```python
from build123d import *

# Parameters (mm, degrees)
SKETCH_R           = 1
SKETCH_W           = 78.96
SKETCH_H           = 50.34
PAD_DEPTH          = 5
SKETCH001_W        = 74.96
SKETCH001_H        = 46.34
PAD001_DEPTH       = 2
SKETCH002_R        = 3
SKETCH002_R_2      = 1
PAD002_DEPTH       = 10
PAD003_DEPTH       = 50
SKETCH004_W        = 40
SKETCH004_H        = 4
POCKET_DEPTH       = 57.001
POCKET_DEPTH_BACK  = -57.001
SKETCH005_R        = 1.5
POCKET001_DEPTH    = 322.817597
POLARPATTERN_COUNT = 4


with BuildPart() as part:
    # Sketch → Pad (new body)
    with BuildSketch(Plane.XY):
        with BuildLine():
            Line((-42.48, 28.17), (-3, 28.17))
            ThreePointArc((3, 28.17), (0, 31.17), (-3, 28.17))
            Line((3, 28.17), (42.48, 28.17))
            Line((42.48, 28.17), (42.48, 3))
            ThreePointArc((42.48, -3), (45.48, 0), (42.48, 3))
            Line((42.48, -3), (42.48, -28.17))
            Line((3, -28.17), (42.48, -28.17))
            ThreePointArc((-3, -28.17), (0, -31.17), (3, -28.17))
            Line((-42.48, -28.17), (-3, -28.17))
            Line((-42.48, -3), (-42.48, -28.17))
            ThreePointArc((-42.48, 3), (-45.48, 0), (-42.48, -3))
            Line((-42.48, 28.17), (-42.48, 3))
        make_face()
        with Locations((42.48, 0)):
            Circle(SKETCH_R, mode=Mode.SUBTRACT)
        with Locations((0, -28.17)):
            Circle(SKETCH_R, mode=Mode.SUBTRACT)
        with Locations((-42.48, 0)):
            Circle(SKETCH_R, mode=Mode.SUBTRACT)
        with Locations((0, 28.17)):
            Circle(SKETCH_R, mode=Mode.SUBTRACT)
        Rectangle(SKETCH_W, SKETCH_H, mode=Mode.SUBTRACT)
    extrude(amount=PAD_DEPTH)

    # Sketch001 → Pad001 (join)
    with BuildSketch(Plane.XY):
        with BuildLine():
            Line((-57, 23.235), (-57, -23.235))
            ThreePointArc((-57, -23.235), (-53.338835, -32.073835), (-44.5, -35.735))
            Line((-44.5, -35.735), (44.5, -35.735))
            ThreePointArc((44.5, -35.735), (53.338835, -32.073835), (57, -23.235))
            Line((57, -23.235), (57, 23.235))
            ThreePointArc((57, 23.235), (53.338835, 32.073835), (44.5, 35.735))
            Line((44.5, 35.735), (-44.5, 35.735))
            ThreePointArc((-44.5, 35.735), (-53.338835, 32.073835), (-57, 23.235))
        make_face()
        Rectangle(SKETCH001_W, SKETCH001_H, mode=Mode.SUBTRACT)
    extrude(amount=PAD001_DEPTH)

    # Sketch002 → Pad002 (join)
    with BuildSketch(Plane.XY):
        with Locations((-46, 24.735)):
            Circle(SKETCH002_R)
        with Locations((-46, 24.735)):
            Circle(SKETCH002_R_2, mode=Mode.SUBTRACT)
        with Locations((46, 24.735)):
            Circle(SKETCH002_R)
        with Locations((46, 24.735)):
            Circle(SKETCH002_R_2, mode=Mode.SUBTRACT)
        with Locations((46, -24.735)):
            Circle(SKETCH002_R)
        with Locations((46, -24.735)):
            Circle(SKETCH002_R_2, mode=Mode.SUBTRACT)
        with Locations((-46, -24.735)):
            Circle(SKETCH002_R)
        with Locations((-46, -24.735)):
            Circle(SKETCH002_R_2, mode=Mode.SUBTRACT)
    extrude(amount=PAD002_DEPTH)

    # Sketch003 → Pad003 (join)
    with BuildSketch(Plane.XY):
        with BuildLine():
            Line((-44.5, 35.735), (44.5, 35.735))
            ThreePointArc((57, 23.235), (53.338835, 32.073835), (44.5, 35.735))
            Line((57, 23.235), (57, -23.235))
            ThreePointArc((44.5, -35.735), (53.338835, -32.073835), (57, -23.235))
            Line((44.5, -35.735), (-44.5, -35.735))
            ThreePointArc((-57, -23.235), (-53.338835, -32.073835), (-44.5, -35.735))
            Line((-57, -23.235), (-57, 23.235))
            ThreePointArc((-44.5, 35.735), (-53.338835, 32.073835), (-57, 23.235))
        make_face()
        with BuildLine():
            Line((-54, 23.235), (-54, -23.235))
            ThreePointArc((-54, -23.235), (-51.217514, -29.952514), (-44.5, -32.735))
            Line((-44.5, -32.735), (44.5, -32.735))
            ThreePointArc((44.5, -32.735), (51.217514, -29.952514), (54, -23.235))
            Line((54, -23.235), (54, 23.235))
            ThreePointArc((54, 23.235), (51.217514, 29.952514), (44.5, 32.735))
            Line((44.5, 32.735), (-44.5, 32.735))
            ThreePointArc((-44.5, 32.735), (-51.217514, 29.952514), (-54, 23.235))
        make_face(mode=Mode.SUBTRACT)
    extrude(amount=PAD003_DEPTH)

    # Sketch004 → Pocket (cut, two sides)
    with BuildSketch(Plane.YZ) as pocket_sk:
        with Locations((0, 48)):
            Rectangle(SKETCH004_W, SKETCH004_H)
    extrude(amount=-POCKET_DEPTH, mode=Mode.SUBTRACT)
    extrude(pocket_sk.sketch, amount=-POCKET_DEPTH_BACK, mode=Mode.SUBTRACT)

    # Sketch005 → Pocket001 (cut, through all)
    with BuildSketch(Plane.XZ):
        with Locations((0, 37.5)):
            Circle(SKETCH005_R)
    pocket001 = extrude(amount=-POCKET001_DEPTH, mode=Mode.SUBTRACT)

    # PolarPattern: Pocket001 ×4 about axis
    polarpattern_axis = Axis((0, 0, 0), (0, 0, 1))
    for i in range(1, POLARPATTERN_COUNT):
        add(pocket001.rotate(polarpattern_axis, i * 360 / POLARPATTERN_COUNT), mode=Mode.SUBTRACT)


solid = part.part
```
The listing builds one solid part. Answer for the finished solid, in the listing's coordinates (mm). A direction names the side the tool comes from. Round coordinates to 2 decimals unless told otherwise and drop trailing zeros. Loops run counter-clockwise (first coordinate to the right, second up) from the corner with the lowest first, then second, coordinate; pieces in that order, holes last. Notation, with made-up numbers: (-3, -11) - (33, -11) arc R20 cw to (33, 7) - close; hole circle Ø5 at (5.5, -11.75). An arc over 180 degrees is marked (long way). Return JSON: item names as keys, results as strings. Group by question number.
1. The part is cut by section B-B on y = -14. Determine the outline of the cut face in (x, z), then the cut area to 3 significant figures.
2. The part is cut by section C-C on z = 13. Determine the outline of the cut face in (x, y) (3 decimals).
3. Each of these flat-tipped pins is pushed along its axis until it touches: P1, Ø1.8, axis at x = 44.5, y = -25, coming from the +Z side; P2, Ø5, axis at x = 0, z = 37.5, coming from the -Y side (3 decimals); P3, Ø2.5, axis at x = 56, y = -7, coming from the +Z side; P4, Ø1, axis at x = 46, y = 24.5, coming from the +Z side. Where does it stop, or does it pass through?
4. The mould has two halves that part along Y. Classify faces 1 (the flat face through (57, 0, 25)), 2 (the cylindrical face through (43.62, -26.56, 5.94)), 3 (the flat face through (-1, -35.735, 25)): pulls with the +Y half, pulls with the -Y half, needs draft (parallel to the pull), parting line crosses it, or undercut.
5. Which of the six approach directions +Z, -Z, +X, -X, +Y, -Y give full straight-line access (tool end or side, diameter ignored) to faces 4 (the flat face through (55, -20, 48)), 5 (the cylindrical face through (0, -34, 36)), 6 (the flat face through (-3, -24, 2))?
6. Consider probe 1 along Y at (x, z) = (0, 3.45) (3 decimals); probe 2 along Y at (x, z) = (21.5, 37) (3 decimals); probe 3 along X at (y, z) = (4.5, 7). Determine where each line is inside the solid, lowest interval first.
7. The part is cut by section A-A on x = -16. Determine the outline of the cut face in (y, z) (3 decimals).
Resolved:
{
 "1": {"outline": "(-57, 0) - (-37.48, 0) - (-37.48, 2) - (-39.48, 2) - (-39.48, 5) - (-42.48, 5) - (-42.48, 2) - (-54, 2) - (-54, 46) - (-57, 46) - close; (37.48, 0) - (57, 0) - (57, 46) - (54, 46) - (54, 2) - (42.48, 2) - (42.48, 5) - (39.48, 5) - (39.48, 2) - (37.48, 2) - close", "area": "360 mm²"},
 "2": {"outline": "(-57, -23.235) arc R12.5 ccw to (-44.5, -35.735) - (44.5, -35.735) arc R12.5 ccw to (57, -23.235) - (57, 23.235) arc R12.5 ccw to (44.5, 35.735) - (-44.5, 35.735) arc R12.5 ccw to (-57, 23.235) - close; hole (-54, -23.235) arc R9.5 ccw to (-44.5, -32.735) - (44.5, -32.735) arc R9.5 ccw to (54, -23.235) - (54, 23.235) arc R9.5 ccw to (44.5, 32.735) - (-44.5, 32.735) arc R9.5 ccw to (-54, 23.235) - close"},
 "3": {"P1": "stops at z = 10", "P2": "stops at y = -35.735", "P3": "stops at z = 46", "P4": "stops at z = 2"},
 "4": {"face 1": "needs draft", "face 2": "undercut", "face 3": "pulls with the -Y half"},
 "5": {"face 4": "+Z, +X, -X", "face 5": "+Y, -Y", "face 6": "+Z"},
 "6": {"probe 1": "y = -35.735 to -32.735, -31.17 to -29.17, -27.17 to -25.17, 25.17 to 27.17, 29.17 to 31.17, 32.735 to 35.735", "probe 2": "y = -35.735 to -32.735, 32.735 to 35.735", "probe 3": "x = -57 to -54, 54 to 57"},
 "7": {"outline": "(-35.735, 0) - (-23.17, 0) - (-23.17, 2) - (-25.17, 2) - (-25.17, 5) - (-28.17, 5) - (-28.17, 2) - (-32.735, 2) - (-32.735, 50) - (-35.735, 50) - close; (23.17, 0) - (35.735, 0) - (35.735, 50) - (32.735, 50) - (32.735, 2) - (28.17, 2) - (28.17, 5) - (25.17, 5) - (25.17, 2) - (23.17, 2) - close"}
}
